```python
from build123d import *

# Parameters (mm, degrees)
SKETCH1_W                      = 35
SKETCH1_H                      = 12.7
BOSS_EXTRUDE1_DEPTH            = 10
CBORE_FOR_M4_SHCS1_AT_2_COUNT  = 2
CBORE_FOR_M4_SHCS1_AT_2_PITCH  = 15
SKETCH4_R                      = 1.7
CUT_EXTRUDE1_DEPTH             = 10
M3_CLEARANCE_HOLE1_D           = 3.6
M3_CLEARANCE_HOLE1_DEPTH       = 5.918450886
M3_CLEARANCE_HOLE1_CSINK_D     = 3.65
M3_CLEARANCE_HOLE1_CSINK_ANGLE = 100
M3_CLEARANCE_HOLE1_TIP         = 1.081549114
SKETCH7_W                      = 5.8
SKETCH7_H                      = 2.71
CUT_EXTRUDE2_DEPTH             = 7.9


with BuildPart() as part:
    # Sketch1 → Boss-Extrude1 (new body)
    with BuildSketch(Plane.XY):
        Rectangle(SKETCH1_W, SKETCH1_H)
    extrude(amount=BOSS_EXTRUDE1_DEPTH)

    # Sketch3 → CBORE for M4 SHCS1 (revolve, cut)
    with BuildSketch(Plane(origin=(12.5, 0, 10), x_dir=(0, -1, 0), z_dir=(1, 0, 0))):
        Polygon((0, 0), (0, 10), (2.4, 10), (2.4, 4), (4, 4), (4, 0.020977491), (4.025, 0), align=None)
    cbore_for_m4_shcs1 = revolve(axis=Axis((12.5, 0, 16.35), (0, 0, -1)), mode=Mode.SUBTRACT)

    # CBORE for M4 SHCS1 at 2: CBORE for M4 SHCS1 ×2
    with Locations(*[(-i * CBORE_FOR_M4_SHCS1_AT_2_PITCH, 0, 0) for i in range(1, CBORE_FOR_M4_SHCS1_AT_2_COUNT)]):
        add(cbore_for_m4_shcs1, mode=Mode.SUBTRACT)

    # Sketch4 → Cut-Extrude1 (cut)
    with BuildSketch(Plane.XY.offset(10)):
        with Locations((-12.5, 0)):
            Circle(SKETCH4_R)
    extrude(amount=-CUT_EXTRUDE1_DEPTH, mode=Mode.SUBTRACT)

    # M3 Clearance Hole1
    with Locations(Plane(origin=(0, 6.35, 0), x_dir=(1, 0, 0), z_dir=(0, 1, 0))):
        with Locations((-12.5, -5)):
            CounterSinkHole(M3_CLEARANCE_HOLE1_D / 2, M3_CLEARANCE_HOLE1_CSINK_D / 2, depth=M3_CLEARANCE_HOLE1_DEPTH, counter_sink_angle=M3_CLEARANCE_HOLE1_CSINK_ANGLE)
            with Locations((0, 0, -(M3_CLEARANCE_HOLE1_DEPTH + M3_CLEARANCE_HOLE1_TIP / 2))):  # 118° drill point
                Cone(0, M3_CLEARANCE_HOLE1_D / 2, M3_CLEARANCE_HOLE1_TIP, mode=Mode.SUBTRACT)

    # Sketch7 → Cut-Extrude2 (cut)
    with BuildSketch(Plane.XY.offset(10)):
        with Locations((-12.5, 4.025)):
            Rectangle(SKETCH7_W, SKETCH7_H)
    extrude(amount=-CUT_EXTRUDE2_DEPTH, mode=Mode.SUBTRACT)


solid = part.part
```
Could you check a few things on this model? Use its own coordinates, in mm. A direction names the side the tool comes from. Coordinates: 2 decimals unless noted, no trailing zeros. Loops run counter-clockwise (first coordinate to the right, second up) from the corner with the lowest first, then second, coordinate; pieces in that order, holes last. Notation, with made-up numbers: M 18.25,-4.75 L 52.25,-4.75 A16 cw 52.25,16.25 Z; hole C 26,85.25 d7. An arc over 180 degrees is marked long. Put each result on its own line as item: value. Start each with the question number.
(1) Will these pins go through, and if not, where does the flat tip stop? P1, Ø2.5, axis at x = 14.5, y = 0, coming from the +Z side; P2, Ø3, axis at x = -12.5, y = 0, coming from the -Z side.
(2) Suppose I cut it at C-C on x = 12.5. Please give me the cut outline in (y, z) (3 decimals).
(3) Suppose I cut it at D-D on z = 5. Please give me the cut outline in (x, y) (3 decimals).
(4) Thinking about a two-plate mould opening in X: for faces 4 (the face through (0, -6.35, 5)), 5 (the face through (-17.5, 0, 5)), 6 (the face through (16.405, 0.867, 8.017)), which applies, pulls with the +X half, pulls with the -X half, needs draft (parallel to the pull), parting line crosses it, or undercut?
(5) I need wall thicknesses on line 1 (Y direction, x = -12.5, z = 2.5); line 2 (Y direction, x = -2.5, z = 9.2); line 3 (Y direction, x = -10, z = 4). Which ranges of each line are inside material? Lowest first, please. Write a range as from..to.
(6) Suppose I cut it at B-B on z = 7.75. Please give me the cut outline in (x, y).
(7) For faces 1 (the face through (-14.163, 1.784, 5.689)), 2 (the face through (15.1, -0.1, 6)), 3 (the face through (10.476, -1.29, 3.042)), which set-ups out of +Z, -Z, +X, -X, +Y, -Y let a thin tool reach every point of the face, with its end or its side?
(8) Suppose I cut it at A-A on x = -12.5. Please give me the cut outline in (y, z) (3 decimals).
Solutions:
1. P1: stops at z = 6
1. P2: passes through
2. outline: M -6.35,0 L -2.4,0 L -2.4,6 L -4,6 L -4,9.979 L -4.025,10 L -6.35,10 Z; M 2.4,0 L 6.35,0 L 6.35,10 L 4.025,10 L 4,9.979 L 4,6 L 2.4,6 Z
3. outline: M -17.5,-6.35 L 17.5,-6.35 L 17.5,6.35 L -10.675,6.35 L -10.7,6.329 L -10.7,5.38 L -9.6,5.38 L -9.6,2.67 L -10.7,2.67 L -10.7,0.432 L -10.836,0.35 A1.7 cw long -14.164,0.35 L -14.3,0.432 L -14.3,2.67 L -15.4,2.67 L -15.4,5.38 L -14.3,5.38 L -14.3,6.329 L -14.325,6.35 L -17.5,6.35 Z; hole C -2.5,0 d4.8; hole C 12.5,0 d4.8
4. face 4: needs draft
4. face 5: pulls with the -X half
4. face 6: undercut
5. line 1: y = -6.35..-1.7, 1.7..2.67, 5.38..6.35
5. line 2: y = -6.35..-4, 4..6.35
5. line 3: y = -6.35..2.67, 5.38..6.35
6. outline: M -17.5,-6.35 L 17.5,-6.35 L 17.5,6.35 L -17.5,6.35 Z; hole M -15.4,2.67 L -9.6,2.67 L -9.6,5.38 L -15.4,5.38 Z; hole C -12.5,0 d3.4; hole C -2.5,0 d8; hole C 12.5,0 d8
7. face 1: +Y
7. face 2: +Z
7. face 3: +Z, -Z
8. outline: M -6.35,0 L -1.7,0 L -1.7,10 L -6.35,10 Z; M 1.7,0 L 6.35,0 L 6.35,3.175 L 6.329,3.2 L 5.38,3.2 L 5.38,2.1 L 2.67,2.1 L 2.67,3.2 L 1.7,3.2 Z; M 1.7,6.8 L 2.67,6.8 L 2.67,10 L 1.7,10 Z; M 5.38,6.8 L 6.329,6.8 L 6.35,6.825 L 6.35,10 L 5.38,10 Z
